from build123d import *

# Parameters (mm, degrees)
SKETCH2_R           = 12.5
BOSS_EXTRUDE1_DEPTH = 30
SKETCH3_R           = 2.5
CUT_EXTRUDE1_DEPTH  = 10
CUT_EXTRUDE2_DEPTH  = 10
CUT_EXTRUDE3_DEPTH  = 5


with BuildPart() as part:
    # Sketch2 → Boss-Extrude1 (new body)
    with BuildSketch(Plane(origin=(0, 0, 0), x_dir=(1, 0, 0), z_dir=(0, 1, 0))):
        with Locations(Location((0, 0, 0), (0, 0, 270))):
            Circle(SKETCH2_R)
    extrude(amount=BOSS_EXTRUDE1_DEPTH)

    # Sketch3 → Cut-Extrude1 (cut)
    with BuildSketch(Plane(origin=(0, 0, 0), x_dir=(-1, 0, 0), z_dir=(0, -1, 0))):
        with Locations(Location((0, 0, 0), (0, 0, 90))):
            Circle(SKETCH3_R)
    extrude(amount=-CUT_EXTRUDE1_DEPTH, mode=Mode.SUBTRACT)

    # Sketch4 → Cut-Extrude2 (cut)
    with BuildSketch(Plane.XZ.offset(-10)):
        with BuildLine():
            Line((2, 1.5), (2, -1.5))
            ThreePointArc((2, -1.5), (-2.5, 0), (2, 1.5))
        make_face()
    extrude(amount=-CUT_EXTRUDE2_DEPTH, mode=Mode.SUBTRACT)

    # Sketch5 → Cut-Extrude3 (cut)
    with BuildSketch(Plane(origin=(0, 30, 0), x_dir=(1, 0, 0), z_dir=(0, 1, 0))):
        Polygon((0, 8.660254038), (-7.5, 4.330127019), (-7.5, -4.330127019), (0, -8.660254038), (7.5, -4.330127019), (7.5, 4.330127019), align=None)
    extrude(amount=-CUT_EXTRUDE3_DEPTH, mode=Mode.SUBTRACT)


solid = part.part
Geometry check sheet. Reference: the model listing, model coordinates, mm. A direction names the side the tool comes from. Give positions to 0.01 mm unless a question says otherwise; leave off trailing zeros. Loops run counter-clockwise (first coordinate to the right, second up) from the corner with the lowest first, then second, coordinate; pieces in that order, holes last. Notation, with made-up numbers: M 62.5,59.5 L 82.5,59.5 A23 cw 82.5,79.5 Z; hole C -16.5,85 d4. An arc over 180 degrees is marked long. Answer as a JSON object with one key per item and string values. Group by question number.
Item 1: Mould release check, pull along X, two halves, no side actions. Record for faces 1 (the flat face through (3.698, 27.535, 6.526)), 2 (the cylindrical face through (3.755, 14.79, 11.923)), 3 (the flat face through (-5, 30, -6)), 4 (the flat face through (0, 25, 0)): pulls with the +X half, pulls with the -X half, needs draft (parallel to the pull), parting line crosses it, or undercut.
Item 2: Sectioned sample at D-D on y = 21.75. Record the boundary of the cut face in (x, z), plus the area to 3 significant figures.
Item 3: Material ranges on L1, parallel to X at y = 5.25, z = 0; L2, parallel to Y at x = 5.5, z = 3.25; L3, parallel to X at y = 15.75, z = 0, recorded low to high.
Item 4: Sectioned sample at A-A on y = 26.5. Record the boundary of the cut face in (x, z).
Item 5: Gauge pin test, flat ends, axial feed: pin 1 (8 mm diameter, centred on x = 6, y = 6.5, fed in from +Z); pin 2 (10 mm diameter, centred on y = 21, z = 8.5, fed in from -X); pin 3 (12 mm diameter, centred on x = 6.5, y = 5, fed in from +Z). Record the tip position at first contact, or that the pin passes through.
Item 6: Access from +Z, -Z, +X, -X, +Y, -Y to the whole of each face (thin tool, end or side, straight path). Record for faces 5 (the flat face through (-3, 0, 0)), 6 (the flat face through (2, 15, 0)), 7 (the flat face through (-3.802, 27.535, 6.465)).
Item 7: Sectioned sample at B-B on z = 0. Record the boundary of the cut face in (x, y), plus the area to 3 significant figures.
Item 8: Sectioned sample at C-C on x = 6.75. Record the boundary of the cut face in (y, z), plus the area to 3 significant figures.
Findings below:
{
 "1": {"face 1": "undercut", "face 2": "parting line crosses it", "face 3": "needs draft", "face 4": "undercut"},
 "2": {"outline": "C 0,0 d25", "area": "491 mm2"},
 "3": {"L1": "-12.5 to -2.5, 2.5 to 12.5", "L2": "0 to 25", "L3": "-12.5 to -2.5, 2 to 12.5"},
 "4": {"outline": "C 0,0 d25; hole M -7.5,-4.33 L 0,-8.66 L 7.5,-4.33 L 7.5,4.33 L 0,8.66 L -7.5,4.33 Z"},
 "5": {"pin 1": "z = 12.34", "pin 2": "x = -12", "pin 3": "z = 12.49"},
 "6": {"face 5": "+Z, -Z, +X, -X, -Y", "face 6": "-Y", "face 7": "+Y"},
 "7": {"outline": "M -12.5,0 L -2.5,0 L -2.5,20 L 2,20 L 2,10 L 2.5,10 L 2.5,0 L 12.5,0 L 12.5,30 L 7.5,30 L 7.5,25 L -7.5,25 L -7.5,30 L -12.5,30 Z", "area": "580 mm2"},
 "8": {"outline": "M 0,-10.52 L 30,-10.52 L 30,-4.76 L 25,-4.76 L 25,4.76 L 30,4.76 L 30,10.52 L 0,10.52 Z", "area": "584 mm2"}
}
